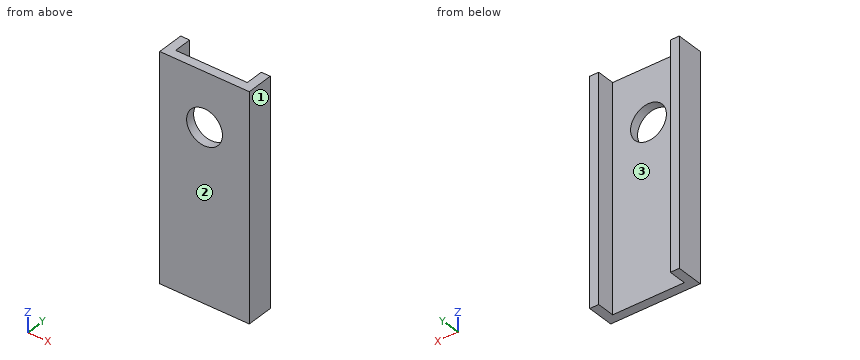
from build123d import *

# Parameters (mm, degrees)
SKETCH052_R      = 2
EXTRUDE049_DEPTH = 5
EXTRUDE048_DEPTH = 25


with BuildPart() as extrude049:
    # Sketch052 → Extrude049 (new body)
    with BuildSketch(Plane.XZ.offset(-35)):
        with Locations((0, 18)):
            Circle(SKETCH052_R)
    extrude(amount=-EXTRUDE049_DEPTH)


with BuildPart() as hook:
    # Sketch051 → Extrude048 (new body)
    with BuildSketch(Plane.XY.offset(-1)):
        Polygon((-5, 40), (-5, 37), (5, 37), (5, 40), (4, 40), (4, 38), (-4, 38), (-4, 40), align=None)
    extrude(amount=EXTRUDE048_DEPTH)

    # Cut041: cut Extrude049
    add(extrude049.part, mode=Mode.SUBTRACT)


solid = hook.part
Could you check a few things on this model? Use its own coordinates, in mm. Face numbers are marked on the shaded views. Coordinates: 2 decimals unless noted, no trailing zeros. Order: outer loops, then holes, each group sorted by start corner. A loop starts at its lowest first (then second) coordinate and runs counter-clockwise, first axis right, second up. Notation, with made-up numbers: (20, -5.5) -> (32, -5.5) arc R9 ccw to (32, 0.5) -> close; hole circle Ø4 at (55, -7). An arc over 180 degrees is marked (long way). One line per item, written item: value. Start each with the question number.
1) Imagine slicing it at A-A on y = 38.8. List the corners of the cut face in (x, z) for me.
2) I'm going to push a flat-ended pin straight in: pin 1 (2.5 mm diameter, centred on x = 1, z = 17, fed in from +Y). Where does the tip first touch, or does it pass through?
3) Imagine slicing it at D-D on z = 13. List the corners of the cut face in (x, y) for me, plus the area to 3 significant figures.
4) If I drill on L1, parallel to Z at x = 0, y = 37.55; L2, parallel to X at y = 39.85, z = 17; L3, parallel to Y at x = -1, z = 0.75, over which ranges is the centre line in solid material (lowest first)? Write a range as [from, to].
5) Imagine slicing it at B-B on z = 18. List the corners of the cut face in (x, y) for me.
6) We'd pull the mould along X, two halves only. Please class the marked faces 1, 2 and 3: +X half, -X half, draft (parallel to the pull), parting line (faces both ways), or undercut.
7) Imagine slicing it at C-C on x = 0. List the corners of the cut face in (y, z) for me, plus the area to 3 significant figures.
Answer list:
1. outline: (-5, -1) -> (-4, -1) -> (-4, 24) -> (-5, 24) -> close; (4, -1) -> (5, -1) -> (5, 24) -> (4, 24) -> close
2. pin 1: stops at y = 38
3. outline: (-5, 37) -> (5, 37) -> (5, 40) -> (4, 40) -> (4, 38) -> (-4, 38) -> (-4, 40) -> (-5, 40) -> close
3. area: 14.0 mm2
4. L1: z = [-1, 16], [20, 24]
4. L2: x = [-5, -4], [4, 5]
4. L3: y = [37, 38]
5. outline: (-5, 37) -> (-2, 37) -> (-2, 38) -> (-4, 38) -> (-4, 40) -> (-5, 40) -> close; (2, 37) -> (5, 37) -> (5, 40) -> (4, 40) -> (4, 38) -> (2, 38) -> close
6. face 1: +X half
6. face 2: draft
6. face 3: undercut
7. outline: (37, -1) -> (38, -1) -> (38, 16) -> (37, 16) -> close; (37, 20) -> (38, 20) -> (38, 24) -> (37, 24) -> close
7. area: 21.0 mm2
